from build123d import *

# Parameters (mm, degrees)
EXTRUDE_390_DEPTH = 10
FILLET_1283_R     = 0.6


with BuildPart() as part:
    # 草图1 → Extrude 390 (new body)
    with BuildSketch(Plane(origin=(0, 0, 0), x_dir=(0, 0, -1), z_dir=(1, 0, 0))):
        Polygon((12, 6.92820323), (12, -6.92820323), (0, -13.856406461), (-12, -6.92820323), (-12, 6.92820323), (0, 13.856406461), align=None)
    extrude(amount=EXTRUDE_390_DEPTH)

    # 草图2 → 凸台-旋转1 (revolve)
    with BuildSketch(Plane.XY, mode=Mode.PRIVATE) as revolve_1_sk:
        Polygon((0, 0), (140, 0), (140, 6.268), (140, 8), (96, 8), (0, 8), align=None)
    revolve(revolve_1_sk.sketch.rotate(Axis((0, 0, 0), (1, 0, 0)), 90), axis=Axis((0, 0, 0), (1, 0, 0)))

    # 草图3 → 切除-旋转1 (revolve, cut)
    with BuildSketch(Plane.XY):
        Polygon((0, 12), (3.958548116, 18.856406461), (3.958548116, 23.856406461), (-10, 23.856406461), (-10, 12), align=None)
    revolve(axis=Axis((0, 0, 0), (1, 0, 0)), mode=Mode.SUBTRACT)

    # 草图4 → 切除-旋转3 (revolve, cut)
    with BuildSketch(Plane.XY, mode=Mode.PRIVATE) as cut_revolve_3_sk:
        Polygon((10, 11.245), (9.2, 11.706880215), (9.2, 13.856406461), (10, 13.856406461), align=None)
    revolve(cut_revolve_3_sk.sketch.rotate(Axis((0, 0, 0), (1, 0, 0)), 90), axis=Axis((0, 0, 0), (1, 0, 0)), mode=Mode.SUBTRACT)

    # Fillet 1283
    fillet_1283_edges = [part.edges().sort_by_distance(p)[0] for p in [
        (10, 0, -8),
    ]]
    fillet(fillet_1283_edges, radius=FILLET_1283_R)


solid = part.part
Design review of the part built by this model. Coordinates are the model's own, in mm. A direction names the side the tool comes from. Give positions to 0.01 mm unless a question says otherwise; leave off trailing zeros. Write each loop counter-clockwise with the first axis right and the second up, starting at its lowest first coordinate (ties: lowest second). Pieces come first, ordered by that corner, then holes. Notation, with made-up numbers: M -3.75,57 L 9.25,57 A27 ccw 9.25,79 Z; hole C 31.25,75.5 d1. An arc over 180 degrees is marked long. Answer as a JSON object with one key per item and string values. Group by question number.
1) Tool access review of faces 1 (the face through (74.39, 7.81, -1.73)), 2 (the face through (4.54, -10.44, 5.92)): name each direction out of +Z, -Z, +X, -X, +Y, -Y from which nothing blocks a thin tool from reaching the whole face with its end or side.
2) For line 1 along X through (y, z) = (5, -10); line 2 along Y through (x, z) = (129, -4); line 3 along Y through (x, z) = (31, -7), list the stretches that pass through material, from the lowest coordinate up.
3) Clearance check with flat-ended pins moving along their axes: pin 1 Ø10 at (x, y) = (79, 5) entering from -Z; pin 2 Ø8 at (y, z) = (8.5, 7) entering from +X; pin 3 Ø2 at (x, z) = (66.5, -3) entering from -Y; pin 4 Ø4 at (x, z) = (34.5, -7) entering from +Y (3 decimals). State where each tip first meets the part, or that it passes through.
4) We need section A-A (x = 33). Give the boundary of the cut face in (y, z), and give its area (3 significant figures).
Answer key:
{
 "1": {"face 1": "+X", "face 2": "+Z, +X, -X, -Y"},
 "2": {"line 1": "x = 0 to 10", "line 2": "y = -6.93 to 6.93", "line 3": "y = -3.87 to 3.87"},
 "3": {"pin 1": "stops at z = -8", "pin 2": "stops at x = 140", "pin 3": "stops at y = -7.75", "pin 4": "stops at y = 6.245"},
 "4": {"outline": "C 0,0 d16", "area": "201 mm²"}
}
